Autodesk Inventor part; units mm, degrees
ref_plane "YZ Plane" through (0, 0, 0) normal (1, 0, 0) x (0, 1, 0)
ref_plane "XZ Plane" through (0, 0, 0) normal (0, 1, 0) x (-1, 0, 0)
ref_plane "XY Plane" through (0, 0, 0) normal (0, 0, 1) x (1, 0, 0)
sketch "Sketch1" plane through (0, 0, 0) normal (0, 1, 0) x (-1, 0, 0)
  line L0 (0, 0) -> (0, 9.525)
  line L1 (0, 9.525) -> (-2.413, 9.525)
  line L2 (-2.413, 9.525) -> (-2.413, 3.2258)
  line L3 (-2.413, 3.2258) -> (-5.2171, 0)
  line L4 (-5.2171, 0) -> (0, 0)
  dimension "d0" = 4.826
  dimension "d2" = 9.525
  dimension "d3" = 41
  dimension "d4" = 3.2258
  dimension "d5" = 5.2172
revolve "Revolution1" add sketch "Sketch1" angle 360 about axis through (0, 0, 0) along (0, 0, 1)
thread "Thread1"
chamfer "Chamfer1" distance 0.508 angle 45 1 edges at (-2.413, 0, 9.525)
sketch "Sketch2" plane through (0, 0, 0) normal (0, 0, -1) x (-1, 0, 0)
  circle A0 centre (0, 0) radius 5.2171
  line L0 (0.9165, -1.5875) -> (-0.9165, -1.5875)
  line L1 (-0.9165, -1.5875) -> (-1.8331, 0)
  line L2 (-1.8331, 0) -> (-0.9165, 1.5875)
  line L3 (-0.9165, 1.5875) -> (0.9165, 1.5875)
  line L4 (0.9165, 1.5875) -> (1.8331, 0)
  line L5 (1.8331, 0) -> (0.9165, -1.5875)
  dimension "d12" = 3.175
extrude "Extrusion1" cut sketch "Sketch2" against normal blind 2.032 contours L0 L1 L2 L3 L4 L5
properties part number "10-32 Flathead x375" material "Steel, Alloy"
Design review of the part built by this model. Coordinates are the model's own, in mm. A direction names the side the tool comes from. Round coordinates to 2 decimals unless told otherwise and drop trailing zeros. Write each loop counter-clockwise with the first axis right and the second up, starting at its lowest first coordinate (ties: lowest second). Pieces come first, ordered by that corner, then holes. Notation, with made-up numbers: (80.5, -1) - (133.5, -1) arc R20 cw to (133.5, 18) - close; hole circle Ø11 at (33, 17). An arc over 180 degrees is marked (long way). Use a Markdown table: item, result. Add a question column.
1. Mouldability with a two-part tool opening along X and no side actions: class faces 3 (the face through (-1.915, 1.468, 6.081)), 4 (the face through (0, 0, 2.032)), 5 (the face through (0, -2, 0)) as +X half, -X half, draft (parallel to the pull), parting line (faces both ways), or undercut.
2. Clearance check with flat-ended pins moving along their axes: pin 1 (3 mm diameter, centred on x = -2.5, z = 3.5, fed in from +Y); pin 2 (2 mm diameter, centred on y = 2, z = 6.5, fed in from -X); pin 3 (5 mm diameter, centred on x = 2, y = 3.5, fed in from +Z) (3 decimals); pin 4 (0.5 mm diameter, centred on x = 0, z = 1, fed in from -Y). State where each tip first meets the part, or that it passes through.
3. We need section B-B (x = 0). State the section outline as (y, z) points (1 decimal).
4. Wall thickness on probe 1 along X at (y, z) = (1, 1); probe 2 along Y at (x, z) = (0.5, 2); probe 3 along X at (y, z) = (-0.5, 1): over which ranges is each line inside the solid? List them lowest first.
5. We need section C-C (z = 8). State the section outline as (x, y) points, then the cut area to 3 significant figures.
6. For faces 1 (the face through (0, 1.588, 1)), 2 (the face through (-0.56, 2.53, 3.02)), list the 3-axis set-ups (+Z, -Z, +X, -X, +Y, -Y) from which the entire face can be reached by the end or side of a thin tool; tool diameter is ignored.
7. We need section A-A (z = 1.75). State the section outline as (x, y) points, then the cut area to 3 significant figures.
Output:
| question | item | result |
|---|---|---|
| 1 | face 3 | parting line |
| 1 | face 4 | undercut |
| 1 | face 5 | draft |
| 2 | pin 1 | stops at y = 2.8 |
| 2 | pin 2 | stops at x = -2.2 |
| 2 | pin 3 | stops at z = 9.525 |
| 2 | pin 4 | stops at y = -4.57 |
| 3 | outline | (-5.2, 0) - (-1.6, 0) - (-1.6, 2) - (1.6, 2) - (1.6, 0) - (5.2, 0) - (2.4, 3.2) - (2.4, 9) - (1.9, 9.5) - (-1.9, 9.5) - (-2.4, 9) - (-2.4, 3.2) - close |
| 4 | probe 1 | x = -4.23 to -1.26, 1.26 to 4.23 |
| 4 | probe 2 | y = -3.44 to -1.59, 1.59 to 3.44 |
| 4 | probe 3 | x = -4.32 to -1.54, 1.54 to 4.32 |
| 5 | outline | circle Ø4.83 at (0, 0) |
| 5 | area | 18.3 mm2 |
| 6 | face 1 | -Z |
| 6 | face 2 | +Z |
| 7 | outline | circle Ø7.39 at (0, 0); hole (-1.83, 0) - (-0.92, -1.59) - (0.92, -1.59) - (1.83, 0) - (0.92, 1.59) - (-0.92, 1.59) - close |
| 7 | area | 34.2 mm2 |
